Autodesk Inventor part; units mm, degrees
ref_plane "YZ Plane" through (0, 0, 0) normal (1, 0, 0) x (0, 1, 0)
ref_plane "XZ Plane" through (0, 0, 0) normal (0, 1, 0) x (-1, 0, 0)
ref_plane "XY Plane" through (0, 0, 0) normal (0, 0, 1) x (1, 0, 0)
sketch "Sketch1" plane through (0, 0, 0) normal (0, 1, 0) x (-1, 0, 0)
  circle A0 centre (0, 0) radius 1.55
  circle A1 centre (0, 0) radius 4.25
  dimension "d0" = 3.1
  dimension "d1" = 8.5
extrude "Extrusion1" add sketch "Sketch1" against normal blind 4
sketch "Sketch2" plane through (0, 0, 0) normal (0, 1, 0) x (1, 0, 0)
  circle A0 centre (0, 0) radius 4.25
extrude "Extrusion2" add sketch "Sketch2" along normal blind 1
sketch "Sketch3" plane through (0, 1, 0) normal (0, 1, 0) x (1, 0, 0)
  circle A0 centre (0, 0) radius 2
  dimension "d6" = 4
extrude "Extrusion3" add sketch "Sketch3" along normal blind 10
fillet "Fillet1" radius 0.5 2 edges at (-2, 1, 0) (-4.25, 1, 0)
chamfer "Chamfer1" distance 1 angle 45 1 edges at (1.55, -4, 0)
properties part number "przycisk"
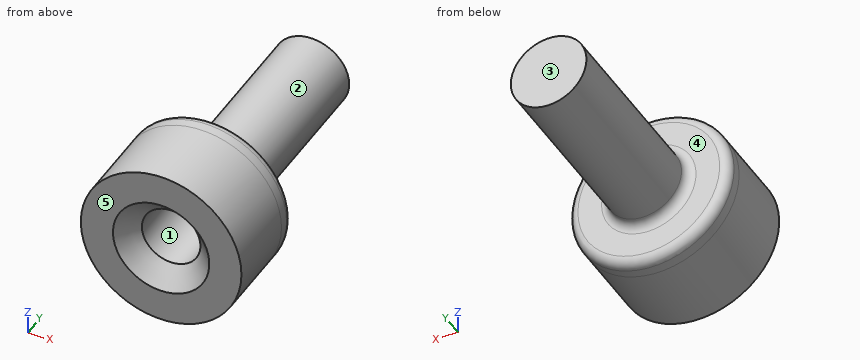
Geometry check sheet. Reference: the model listing, model coordinates, mm. Face numbers are marked on the shaded views. A direction names the side the tool comes from. Round coordinates to 2 decimals unless told otherwise and drop trailing zeros. Write each loop counter-clockwise with the first axis right and the second up, starting at its lowest first coordinate (ties: lowest second). Pieces come first, ordered by that corner, then holes. Notation, with made-up numbers: (64.25, 27) -> (117.25, 27) arc R19 cw to (117.25, 39) -> close; hole circle Ø7 at (-34.75, 67). An arc over 180 degrees is marked (long way). One line per item, written item: value. Start each with the question number.
(1) Go/stop test with flat-tipped pins: pin 1 Ø1 at (x, y) = (2, 8) entering from -Z; pin 2 Ø1 at (y, z) = (6.5, -2) entering from +X; pin 3 Ø5 at (y, z) = (5.5, -1) entering from +X. Record where each tip stops, or that it passes through.
(2) Access from +Z, -Z, +X, -X, +Y, -Y to the whole of each face (thin tool, end or side, straight path). Record for the marked faces 4 and 5.
(3) Cross-section at D-D, the plane y = 0.75. Record the cut outline in (x, z), and give its area (3 significant figures).
(4) Draft check along Z on the marked faces 1, 2 and 3. Enter one of: +Z half, -Z half, draft (parallel to the pull), parting line (faces both ways), or undercut.
(5) Cross-section at B-B, the plane y = -0.75. Record the cut outline in (x, z).
(6) Cross-section at C-C, the plane y = 3.25. Record the cut outline in (x, z), and give its area (3 significant figures).
(7) Cross-section at A-A, the plane x = 0. Record the cut outline in (y, z), and give its area (3 significant figures).
(8) Scan lines: line 1 (Z direction, x = 0, y = -0.8); line 2 (Z direction, x = 0, y = 1.75); line 3 (Y direction, x = -0.75, z = 0). Record each from-to range of solid material in increasing order. Write a range as [from, to].
Answer:
1. pin 1: z = -1.32
1. pin 2: x = 1.32
1. pin 3: x = 2
2. face 4: +Y
2. face 5: +Z, -Z, +X, -X, -Y
3. outline: circle Ø8.37 at (0, 0)
3. area: 55.0 mm²
4. face 1: undercut
4. face 2: parting line
4. face 3: draft
5. outline: circle Ø8.5 at (0, 0); hole circle Ø3.1 at (0, 0)
6. outline: circle Ø4 at (0, 0)
6. area: 12.6 mm²
7. outline: (-4, -4.25) -> (0.5, -4.25) arc R0.5 ccw to (1, -3.75) -> (1, -2.5) arc R0.5 cw to (1.5, -2) -> (11, -2) -> (11, 2) -> (1.5, 2) arc R0.5 cw to (1, 2.5) -> (1, 3.75) arc R0.5 ccw to (0.5, 4.25) -> (-4, 4.25) -> (-4, 2.55) -> (-3, 1.55) -> (0, 1.55) -> (0, -1.55) -> (-3, -1.55) -> (-4, -2.55) -> close
7. area: 69.1 mm²
8. line 1: [-4.25, -1.55], [1.55, 4.25]
8. line 2: [-2, 2]
8. line 3: [0, 11]
